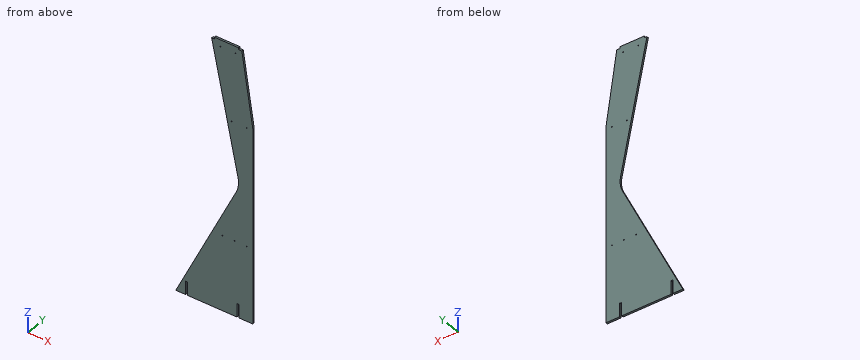
```python
from build123d import *

# Parameters (mm, degrees)
F1_DEPTH = 3.15
F2_W     = 30.610543
F2_H     = 6
F2_W_2   = 33.654636
F2_W_3   = 6.6
F2_H_2   = 45
F3_DEPTH = 6.301
F5_D     = 3


with BuildPart() as f1:
    # F0 (on Front) → F1 (new body, symmetric)
    with BuildSketch(Plane.XZ):
        with BuildLine():
            Line((90, 450), (-10, 450))
            Line((-10, 450), (78.390962, 15.964244))
            ThreePointArc((78.390962, 15.964244), (79.395078, -9.81945), (72.139537, -34.581603))
            Line((72.139537, -34.581603), (-127, -450))
            Line((-127, -450), (127, -450))
            Line((127, -450), (127, 200))
            Line((127, 200), (90, 450))
        make_face()
    extrude(amount=F1_DEPTH, both=True)

    # F2 (on face) → F3 (cut, through all)
    with BuildSketch(Plane.XZ.offset(3.15)):
        with Locations((-15.305271, 447)):
            Rectangle(F2_W, F2_H)
        with Locations((96.827318, 447)):
            Rectangle(F2_W_2, F2_H)
        with Locations((-91.615785, -427.5)):
            Rectangle(F2_W_3, F2_H_2)
        with Locations((77.765864, -427.5)):
            Rectangle(F2_W_3, F2_H_2)
    extrude(amount=-F3_DEPTH, mode=Mode.SUBTRACT)

    # F5 (through all)
    with Locations(Plane.XZ.offset(3.15)):
        with Locations((20, 427.3), (70, 427.3), (107, 194), (57, 194), (107, -200), (67, -200), (27, -200)):
            Hole(F5_D / 2)


solid = f1.part
```
Read the model definition and answer for the solid it produces. Units are mm, in the model's axes. Give positions to 0.01 mm unless a question says otherwise; leave off trailing zeros. Write each loop counter-clockwise with the first axis right and the second up, starting at its lowest first coordinate (ties: lowest second). Pieces come first, ordered by that corner, then holes. Notation, with made-up numbers: M 68,18 L 87,18 A12 cw 87,25 Z; hole C 74,36 d2. An arc over 180 degrees is marked long. Put each result on its own line as item: value. Start each with the question number.
1. The part is cut by section D-D, the plane x = -28. Give the vertices of the cut face in (y, z), and give its area (3 significant figures).
2. The part is cut by section C-C, the plane z = 144. Give the vertices of the cut face in (x, y), and give its area (3 significant figures).
3. The part is cut by section A-A, the plane y = -0.5. Give the vertices of the cut face in (x, z).
4. Consider line 1 along X through (y, z) = (1.25, -200); line 2 along X through (y, z) = (1, 427.3); line 3 along X through (y, z) = (1, 194). Determine where each line is inside the solid, lowest interval first.
5. The part is cut by section B-B, the plane x = 43. Give the vertices of the cut face in (y, z), and give its area (3 significant figures).
6. Each of these flat-tipped pins is pushed along its axis until it touches: pin 1 Ø1.9 at (x, y) = (-92, -0.5) entering from -Z; pin 2 Ø2.5 at (x, z) = (70, 427.3) entering from -Y; pin 3 Ø1.5 at (y, z) = (2.5, 78.5) entering from -X. Where does it stop, or does it pass through?
Final values:
1. outline: M -3.15,-450 L 3.15,-450 L 3.15,-243.48 L -3.15,-243.48 Z
1. area: 1,300 mm²
2. outline: M 52.32,-3.15 L 127,-3.15 L 127,3.15 L 52.32,3.15 Z
2. area: 471 mm²
3. outline: M -127,-450 L -94.92,-450 L -94.92,-405 L -88.32,-405 L -88.32,-450 L 74.47,-450 L 74.47,-405 L 81.07,-405 L 81.07,-450 L 127,-450 L 127,200 L 90.89,444 L 80,444 L 80,450 L 0,450 L 0,444 L -8.78,444 L 78.39,15.96 A80 cw 72.14,-34.58 Z; hole C 20,427.3 d3; hole C 27,-200 d3; hole C 57,194 d3; hole C 67,-200 d3; hole C 70,427.3 d3; hole C 107,-200 d3; hole C 107,194 d3
4. line 1: x = -7.16 to 25.5, 28.5 to 65.5, 68.5 to 105.5, 108.5 to 127
4. line 2: x = -5.38 to 18.5, 21.5 to 68.5, 71.5 to 93.36
4. line 3: x = 42.13 to 55.5, 58.5 to 105.5, 108.5 to 127
5. outline: M -3.15,-450 L 3.15,-450 L 3.15,-95.37 L -3.15,-95.37 Z; M -3.15,189.75 L 3.15,189.75 L 3.15,450 L -3.15,450 Z
5. area: 3,870 mm²
6. pin 1: stops at z = -405
6. pin 2: passes through
6. pin 3: stops at x = 65.5
